For this review, use the dimensioned drawing (mm, ordinates from the lowest corner) and the shaded views. A direction names the side the tool comes from. Coordinates: 2 decimals unless noted, no trailing zeros. Write each loop counter-clockwise with the first axis right and the second up, starting at its lowest first coordinate (ties: lowest second). Pieces come first, ordered by that corner, then holes.
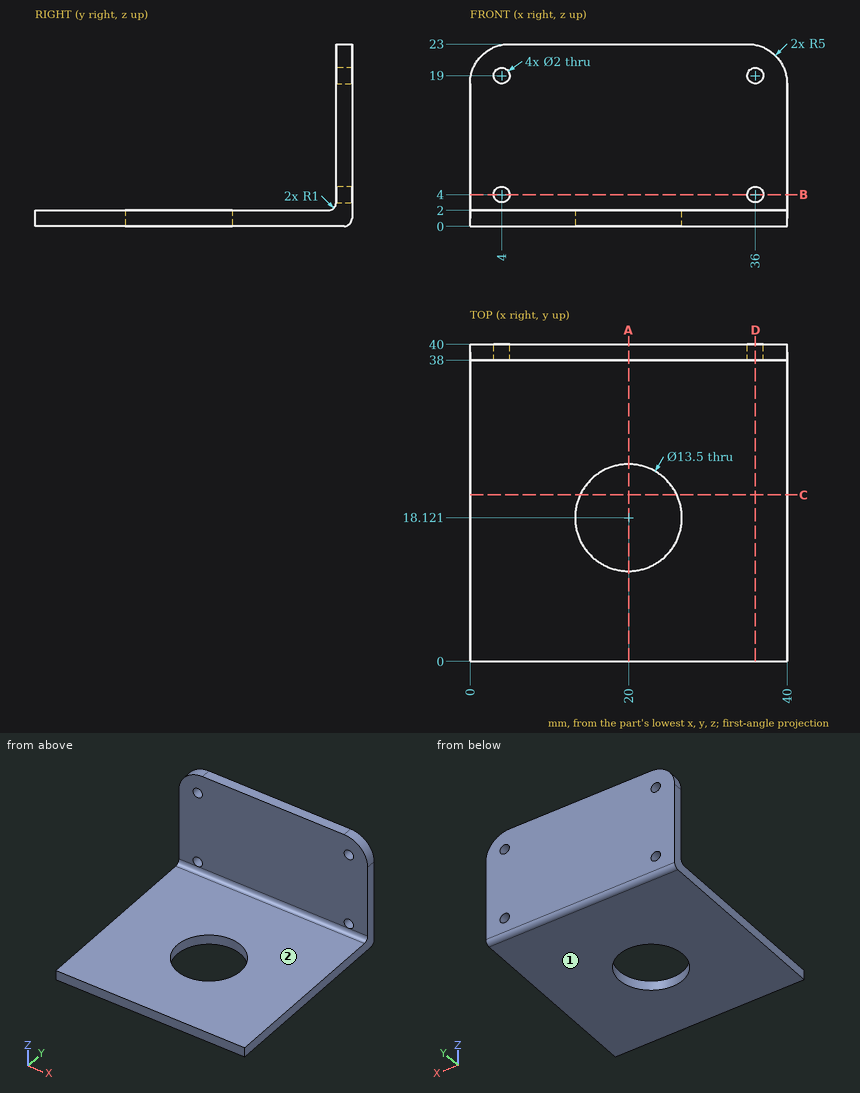
Item 1: Machinability: for the marked faces 1 and 2, which of the approach directions +Z, -Z, +X, -X, +Y, -Y give a long, thin tool a straight path to every point of the face, cutting with its end or side? Answer none if there is none.
Solved:
face 1: -Z, +X, -X, +Y, -Y
face 2: +Z, +X, -X, -Y
Item 2: To check wall thickness, follow line 1 along X through (y, z) = (39.55, 4); line 2 along X through (y, z) = (39.35, 19); line 3 along Y through (x, z) = (20, 1.4). State the ranges of each line that lie inside material, in increasing order.
Solved:
line 1: x = 0 to 3, 5 to 35, 37 to 40
line 2: x = 0.1 to 3, 5 to 35, 37 to 39.9
line 3: y = 0 to 11.37, 24.87 to 40
Item 3: Take a section at C-C, the plane y = 21. Write out the cut boundary in (x, z) (1 decimal).
Solved:
outline: (0, 0) - (13.9, 0) - (13.9, 2) - (0, 2) - close; (26.1, 0) - (40, 0) - (40, 2) - (26.1, 2) - close
Item 4: Take a section at B-B, the plane z = 4. Write out the cut boundary in (x, y), plus the area to 3 significant figures.
Solved:
outline: (0, 38) - (3, 38) - (3, 40) - (0, 40) - close; (5, 38) - (35, 38) - (35, 40) - (5, 40) - close; (37, 38) - (40, 38) - (40, 40) - (37, 40) - close
area: 72.0 mm2
Item 5: Take a section at D-D, the plane x = 36. Count the separate pieces of the cut face and the enclosed holes in it, plus the area to 3 significant figures.
Solved:
separate pieces: 3
enclosed holes: 0
area: 114 mm2
Item 6: For pin 1 (8 mm diameter, centred on x = 12.5, y = 9, fed in from +Z); pin 2 (1 mm diameter, centred on x = 13.5, z = 18.5, fed in from -Y); pin 3 (3 mm diameter, centred on x = 36, z = 4, fed in from -Y), all flat-tipped, find the tip position at first contact; note any pin that passes through.
Solved:
pin 1: stops at z = 2
pin 2: stops at y = 38
pin 3: stops at y = 37.87
Item 7: Take a section at A-A, the plane x = 20. Write out the cut boundary in (y, z), plus the area to 3 significant figures.
Solved:
outline: (0, 0) - (11.37, 0) - (11.37, 2) - (0, 2) - close; (24.87, 0) - (39, 0) arc R1 ccw to (40, 1) - (40, 23) - (38, 23) - (38, 3) arc R1 cw to (37, 2) - (24.87, 2) - close
area: 95.0 mm2
